from build123d import *

# Parameters (mm, degrees)
BOSS_EXTRUDE1_DEPTH = 0.8
CHAMFER1_SIZE       = 0.2
FILLET1_R           = 1
FILLET2_R           = 0.5


with BuildPart() as part:
    # Sketch1 → Boss-Extrude1 (new body)
    with BuildSketch(Plane(origin=(0, 0, 0), x_dir=(1, 0, 0), z_dir=(0, 1, 0))):
        with BuildLine():
            Line((9.1, 0), (21.1, 0))
            Line((21.1, 0), (21.1, 4))
            Line((21.1, 4), (22.2, 4))
            Line((22.2, 4), (22.2, 0))
            Line((22.2, 0), (28.9, 0))
            Line((28.9, 0), (28.9, 4))
            Line((28.9, 4), (38, 4))
            Line((38, 4), (38, 42.7))
            ThreePointArc((38, 42.7), (36.7, 44), (38, 45.3))
            Line((38, 45.3), (38, 65))
            Line((38, 65), (0, 65))
            Line((0, 65), (0, 45.3))
            ThreePointArc((0, 45.3), (1.3, 44), (0, 42.7))
            Line((0, 42.7), (0, 4))
            Line((0, 4), (9.1, 4))
            Line((9.1, 4), (9.1, 0))
        make_face()
    extrude(amount=BOSS_EXTRUDE1_DEPTH)

    # Chamfer1
    chamfer1_edges = [part.edges().sort_by_distance(p)[0] for p in [
        (25.55, 0, 0),
        (15.1, 0, 0),
        (15.1, 0.8, 0),
        (25.55, 0.8, 0),
    ]]
    chamfer(chamfer1_edges, length=CHAMFER1_SIZE)

    # Fillet1
    fillet1_edges = [part.edges().sort_by_distance(p)[0] for p in [
        (38, 0.4, -4),
        (28.9, 0.4, -4),
        (9.1, 0.4, -4),
        (0, 0.4, -4),
    ]]
    fillet(fillet1_edges, radius=FILLET1_R)

    # Fillet2
    fillet2_edges = [part.edges().sort_by_distance(p)[0] for p in [
        (22.2, 0.4, -4),
        (21.1, 0.4, -4),
    ]]
    fillet(fillet2_edges, radius=FILLET2_R)


solid = part.part
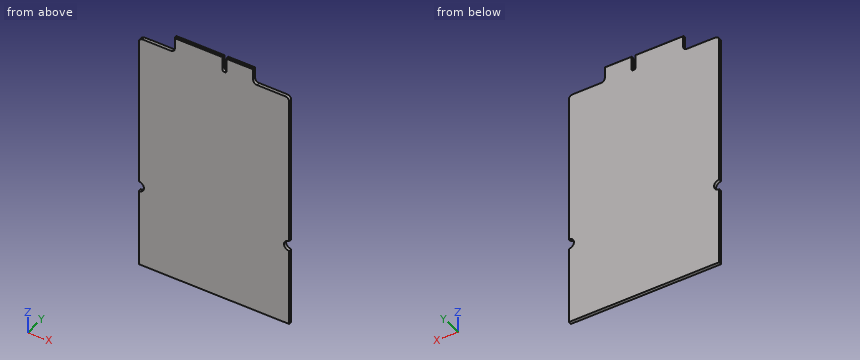
Read the model definition and answer for the solid it produces. Units are mm, in the model's axes. Coordinates: 2 decimals unless noted, no trailing zeros. Write each loop counter-clockwise with the first axis right and the second up, starting at its lowest first coordinate (ties: lowest second). Pieces come first, ordered by that corner, then holes. Notation, with made-up numbers: M -3.75,-37 L 19.25,-37 A15 cw 19.25,-16 Z; hole C 20.5,31.25 d7. An arc over 180 degrees is marked long. Use a Markdown table: item, result.
Q1. Straight lines are drawn through the part: L1, parallel to Z at x = 34, y = 0.75; L2, parallel to Z at x = 15, y = 0.75. For each, find the intervals that lie inside material, in ascending order. Write a range as [from, to].
Answer block:
| item | result |
|---|---|
| L1 | z = [-65, -4] |
| L2 | z = [-65, -0.15] |
Q2. The part is cut by section A-A, the plane y = 0.35. Write down the section's boundary in (x, z).
Answer block:
| item | result |
|---|---|
| outline | M 0,-65 L 38,-65 L 38,-45.3 A1.3 cw 38,-42.7 L 38,-5 A1 ccw 37,-4 L 29.9,-4 A1 cw 28.9,-3 L 28.9,0 L 22.2,0 L 22.2,-3.5 A0.5 cw 21.7,-4 L 21.6,-4 A0.5 cw 21.1,-3.5 L 21.1,0 L 9.1,0 L 9.1,-3 A1 cw 8.1,-4 L 1,-4 A1 ccw 0,-5 L 0,-42.7 A1.3 cw 0,-45.3 Z |
Q3. The part is cut by section B-B, the plane x = 35. Write down the section's boundary in (y, z).
Answer block:
| item | result |
|---|---|
| outline | M 0,-65 L 0.8,-65 L 0.8,-4 L 0,-4 Z |
Q4. The part is cut by section C-C, the plane z = -44. Write down the section's boundary in (x, y), then the cut area to 3 significant figures.
Answer block:
| item | result |
|---|---|
| outline | M 1.3,0 L 36.7,0 L 36.7,0.8 L 1.3,0.8 Z |
| area | 28.3 mm2 |
